```python
from build123d import *

# Parameters (mm, degrees)
SKETCH1_W                   = 133.35
SKETCH1_H                   = 47.625
BOSS_EXTRUDE1_DEPTH         = 15.8623
CUT_EXTRUDE2_START          = -23.8125
SKETCH2_R                   = 8.3312
CUT_EXTRUDE2_DEPTH          = 133.35
CUT_EXTRUDE4_START          = -23.8125
SKETCH3_R                   = 12.7
CUT_EXTRUDE4_DEPTH          = 15.875
CUT_EXTRUDE6_START          = -15.8623
SKETCH4_R                   = 10.3124
CUT_EXTRUDE6_DEPTH          = 89.417129905
F_3_4_16_TAPPED_HOLE1_D     = 17.4625
F_3_4_16_TAPPED_HOLE1_DEPTH = 31.7246
F_3_4_16_TAPPED_HOLE1_TIP   = 5.24626428
CHAMFER1_SIZE               = 1.5875


with BuildPart() as part:
    # Sketch1 → Boss-Extrude1 (new, symmetric)
    with BuildSketch(Plane(origin=(0, 0, 0), x_dir=(1, 0, 0), z_dir=(0, 1, 0))):
        Rectangle(SKETCH1_W, SKETCH1_H)
    extrude(amount=BOSS_EXTRUDE1_DEPTH, both=True)

    # Sketch2 → Cut-Extrude2 (cut)
    with BuildSketch(Plane.XY.offset(CUT_EXTRUDE2_START)):
        with Locations(Location((-50.8, -0.0127, 0), (0, 0, 180))):
            Circle(SKETCH2_R)
        with Locations(Location((50.8, -0.0127, 0), (0, 0, 180))):
            Circle(SKETCH2_R)
    extrude(amount=CUT_EXTRUDE2_DEPTH, mode=Mode.SUBTRACT)

    # Sketch3 → Cut-Extrude4 (cut)
    with BuildSketch(Plane.XY.offset(CUT_EXTRUDE4_START)):
        with Locations((-50.8, -0.0127)):
            Circle(SKETCH3_R)
        with Locations((50.8, -0.0127)):
            Circle(SKETCH3_R)
    extrude(amount=CUT_EXTRUDE4_DEPTH, mode=Mode.SUBTRACT)

    # Sketch4 → Cut-Extrude6 (cut, through all)
    with BuildSketch(Plane(origin=(0, 0, 0), x_dir=(1, 0, 0), z_dir=(0, 1, 0)).offset(CUT_EXTRUDE6_START)):
        with Locations(Location((25.4, 7.9375, 0), (0, 0, 270))):
            Circle(SKETCH4_R)
    extrude(amount=CUT_EXTRUDE6_DEPTH, mode=Mode.SUBTRACT)

    # 3/4-16 Tapped Hole1
    with Locations(Plane(origin=(0, -15.8623, 0), x_dir=(-1, 0, 0), z_dir=(0, -1, 0))):
        with Locations((25.4, 7.9375)):
            Hole(F_3_4_16_TAPPED_HOLE1_D / 2, depth=F_3_4_16_TAPPED_HOLE1_DEPTH)
            with Locations((0, 0, -(F_3_4_16_TAPPED_HOLE1_DEPTH + F_3_4_16_TAPPED_HOLE1_TIP / 2))):  # 118° drill point
                Cone(0, F_3_4_16_TAPPED_HOLE1_D / 2, F_3_4_16_TAPPED_HOLE1_TIP, mode=Mode.SUBTRACT)

    # Chamfer1
    chamfer1_edges = [part.edges().sort_by_distance(p)[0] for p in [
        (-66.675, 15.8623, 0),
        (0, 15.8623, 23.8125),
        (66.675, 15.8623, 0),
        (0, -15.8623, 23.8125),
        (-66.675, -15.8623, 0),
        (66.675, -15.8623, 0),
    ]]
    chamfer(chamfer1_edges, length=CHAMFER1_SIZE)


solid = part.part
```
Geometry: final body of the model. Coordinates: model frame, mm. A direction names the side the tool comes from. Give positions to 0.01 mm unless a question says otherwise; leave off trailing zeros. Loops run counter-clockwise (first coordinate to the right, second up) from the corner with the lowest first, then second, coordinate; pieces in that order, holes last. Notation, with made-up numbers: (-18.5, 3) -> (25.5, 3) arc R20 ccw to (25.5, 40) -> close; hole circle Ø1 at (66, 61). An arc over 180 degrees is marked (long way). Return JSON: item names as keys, results as strings.
Item 1: Section B-B, the plane z = -1.5. Output: boundary loops of the cut face in (x, y) (1 decimal), plus the area to 3 significant figures.
Filled in:
{"outline": "(-66.7, -14.3) -> (-65.1, -15.9) -> (-31.3, -15.9) -> (-31.3, 15.9) -> (-65.1, 15.9) -> (-66.7, 14.3) -> close; (-19.5, -15.9) -> (17.3, -15.9) -> (17.3, 15.9) -> (-19.5, 15.9) -> close; (33.5, -15.9) -> (65.1, -15.9) -> (66.7, -14.3) -> (66.7, 14.3) -> (65.1, 15.9) -> (33.5, 15.9) -> close; hole circle Ø16.7 at (-50.8, 0); hole circle Ø16.7 at (50.8, 0)", "area": "2,900 mm^2"}
Item 2: Access query for faces 4 (the cylindrical face through (-58.746, -2.515, 7.715)), 5 (the cylindrical face through (38.112, 0.546, -15.986)). Directions: +Z, -Z, +X, -X, +Y, -Y. A direction counts if a zero-diameter tool reaches every point of the face in a straight line with its end or side. Return the directions, or none.
Filled in:
{"face 4": "+Z, -Z", "face 5": "-Z"}
Item 3: Line query: line 1 (Y direction, x = -50.8, z = 4); line 2 (Z direction, x = 25.4, y = 5.5); line 3 (X direction, y = 2, z = 11.5) (3 decimals). Output: solid intervals per line, ascending.
Filled in:
{"line 1": "-15.86 to -8.34, 8.32 to 15.86", "line 2": "-23.81 to -18.25, 2.37 to 23.81", "line 3": "-66.675 to -58.884, -42.716 to 42.716, 58.884 to 66.675"}
Item 4: Pin query (flat end, axial travel): P1, Ø12.5, axis at x = -56.5, y = 0, coming from the -Z side. Return the tip coordinate at first contact, or that it passes through.
Filled in:
{"P1": "z = -7.94"}
Item 5: Section A-A, the plane x = 50.8. Output: boundary loops of the cut face in (y, z) (1 decimal), plus the area to 3 significant figures.
Filled in:
{"outline": "(-15.9, -23.8) -> (-12.7, -23.8) -> (-12.7, -7.9) -> (-8.3, -7.9) -> (-8.3, 23.8) -> (-14.3, 23.8) -> (-15.9, 22.2) -> close; (8.3, -7.9) -> (12.7, -7.9) -> (12.7, -23.8) -> (15.9, -23.8) -> (15.9, 22.2) -> (14.3, 23.8) -> (8.3, 23.8) -> close", "area": "576 mm^2"}
Item 6: Mould query, pull axis X, two halves, no side actions, for faces 1 (the flat face through (-1, -15.862, -1)), 2 (the flat face through (-66.675, 0, 0)), 3 (the cylindrical face through (-38.686, 3.802, -15.986)). Classes: released by +X, released by -X, zero draft, split by the parting line, or undercut.
Filled in:
{"face 1": "zero draft", "face 2": "released by -X", "face 3": "undercut"}
Item 7: Section C-C, the plane y = 6.5. Output: boundary loops of the cut face in (x, z) (1 decimal), plus the area to 3 significant figures.
Filled in:
{"outline": "(-66.7, -23.8) -> (-61.7, -23.8) -> (-61.7, -7.9) -> (-56, -7.9) -> (-56, 23.8) -> (-66.7, 23.8) -> close; (-45.6, -7.9) -> (-39.9, -7.9) -> (-39.9, -23.8) -> (39.9, -23.8) -> (39.9, -7.9) -> (45.6, -7.9) -> (45.6, 23.8) -> (-45.6, 23.8) -> close; (56, -7.9) -> (61.7, -7.9) -> (61.7, -23.8) -> (66.7, -23.8) -> (66.7, 23.8) -> (56, 23.8) -> close; hole circle Ø17.5 at (-25.4, -7.9); hole circle Ø20.6 at (25.4, -7.9)", "area": "4,430 mm^2"}
Item 8: Section D-D, the plane z = 10.5. Output: boundary loops of the cut face in (x, y) (1 decimal).
Filled in:
{"outline": "(-66.7, -14.3) -> (-65.1, -15.9) -> (65.1, -15.9) -> (66.7, -14.3) -> (66.7, 14.3) -> (65.1, 15.9) -> (-65.1, 15.9) -> (-66.7, 14.3) -> close; hole circle Ø16.7 at (-50.8, 0); hole circle Ø16.7 at (50.8, 0)"}
